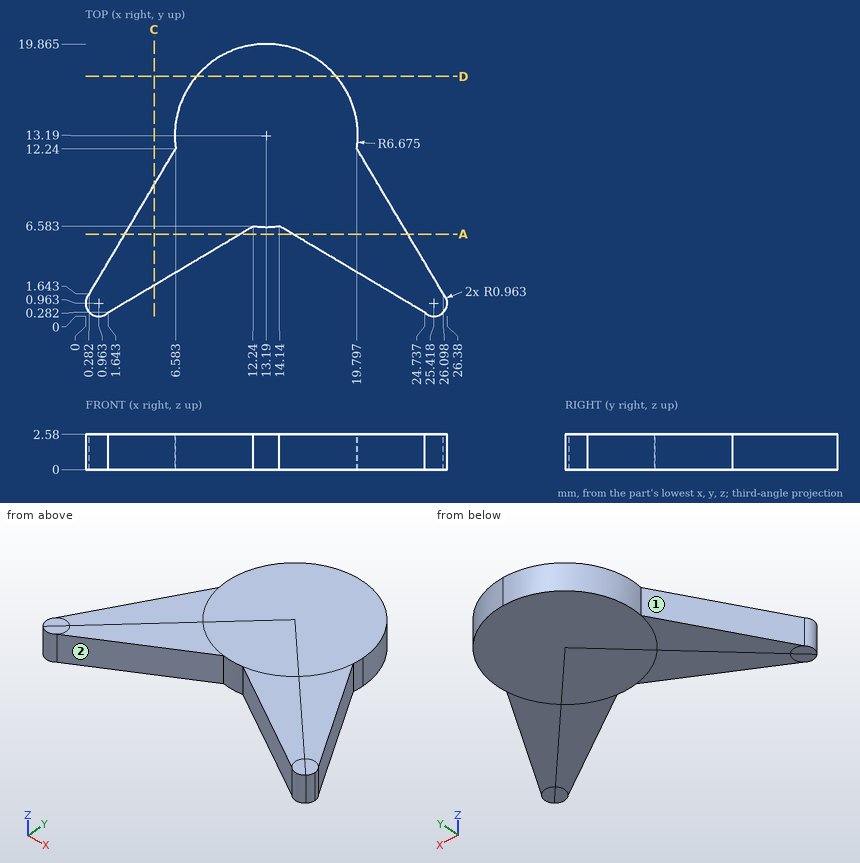
Verification items for this drawing (mm, ordinates from the low corner). Give positions to 0.01 mm unless a question says otherwise; leave off trailing zeros. Write each loop counter-clockwise with the first axis right and the second up, starting at its lowest first coordinate (ties: lowest second). Pieces come first, ordered by that corner, then holes. Notation, with made-up numbers: (-9, -5.75) -> (38, -5.75) arc R16 ccw to (38, 1.25) -> close; hole circle Ø8 at (77, 43.25). An arc over 180 degrees is marked (long way). Use one line per item in the form item = value.
Item 1: Mould release check, pull along X, two halves, no side actions. Record for the marked faces 1 and 2: released by +X, released by -X, zero draft, split by the parting line, or undercut.
Results list:
face_1 = released by -X
face_2 = undercut
Item 2: Depth check by flat-ended pin: pin 1 Ø1.5 at (y, z) = (10.5, 1) entering from +X; pin 2 Ø1.5 at (y, z) = (9, 1) entering from +X; pin 3 Ø2 at (x, y) = (16, 6) entering from -Z; pin 4 Ø1.5 at (x, z) = (16, 2) entering from +Y. Enter the tip coordinate at first touch or a pass-through.
Results list:
pin_1 = 21.28
pin_2 = 22.17
pin_3 = 0
pin_4 = 19.54
Item 3: Sectioned sample at C-C on x = 5. Enter the section's corners in (y, z).
Results list:
outline = (2.28, 0) -> (9.58, 0) -> (9.58, 2.58) -> (2.28, 2.58) -> close
Item 4: Sectioned sample at A-A on y = 6. Enter the section's corners in (x, z).
Results list:
outline = (2.87, 0) -> (11.26, 0) -> (11.26, 2.58) -> (2.87, 2.58) -> close; (15.12, 0) -> (23.51, 0) -> (23.51, 2.58) -> (15.12, 2.58) -> close
Item 5: Scan lines: line 1 (Y direction, x = 4.5, z = 0.5) (1 decimal); line 2 (X direction, y = 7.25, z = 2.2) (1 decimal); line 3 (X direction, y = 18, z = 1.5) (1 decimal). Record each from-to range of solid material in increasing order.
Results list:
line_1 = 2 to 8.7
line_2 = 3.6 to 22.8
line_3 = 8.6 to 17.8
Item 6: Sectioned sample at D-D on y = 17.5. Enter the section's corners in (x, z).
Results list:
outline = (8.09, 0) -> (18.29, 0) -> (18.29, 2.58) -> (8.09, 2.58) -> close
